Geometry: final body of the model. Coordinates: model frame, mm. Face numbers are marked on the shaded views. Round coordinates to 2 decimals unless told otherwise and drop trailing zeros. Loops run counter-clockwise (first coordinate to the right, second up) from the corner with the lowest first, then second, coordinate; pieces in that order, holes last. Notation, with made-up numbers: M 33,9.25 L 79,9.25 A17 ccw 79,14.25 Z; hole C -9.5,27.25 d2. An arc over 180 degrees is marked long. Answer as a JSON object with one key per item and string values.
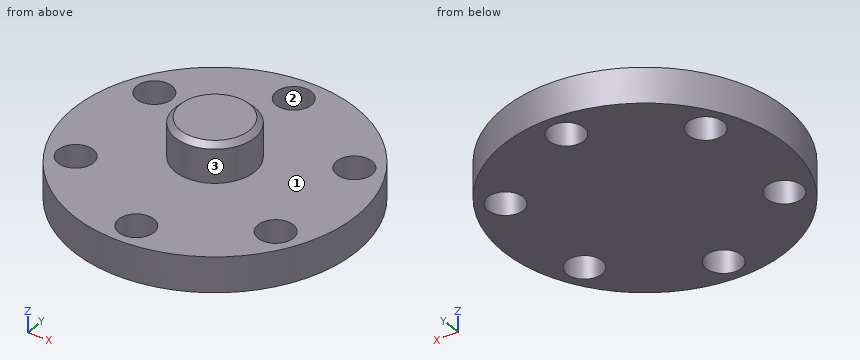
```python
from build123d import *

# Parameters (mm, degrees)
SKETCH1_R               = 80
BASE_EXTRUDE_DEPTH      = 20
CHAMFER1_SIZE           = 3
HOLE_WIZARD_20_0_20_1_D = 20
CIRPATTERN2_COUNT       = 6


with BuildPart() as part:
    # Sketch1 → Base-Extrude (new body)
    with BuildSketch(Plane.XY):
        Circle(SKETCH1_R)
    extrude(amount=BASE_EXTRUDE_DEPTH)

    # Sketch2 → Boss-Revolve1 (revolve)
    with BuildSketch(Plane(origin=(0, 0, 0), x_dir=(1, 0, 0), z_dir=(0, 1, 0))):
        Polygon((-10, -20), (-10, -23), (-22.5, -23), (-22.5, -45), (0, -45), (0, -20), align=None)
    revolve(axis=Axis((0, 0, 0), (0, 0, 1)))

    # Chamfer1
    chamfer1_edges = [part.edges().sort_by_distance(p)[0] for p in [
        (22.5, 0, 45),
    ]]
    chamfer(chamfer1_edges, length=CHAMFER1_SIZE)

    # Ø20.0 (20) 直徑孔1 (through all)
    with Locations(Plane(origin=(0, 65, 20), x_dir=(1, 0, 0), z_dir=(0, 0, 1))):
        with Locations((0, 0)):
            hole_wizard_20_0_20_1 = Hole(HOLE_WIZARD_20_0_20_1_D / 2)

    # CirPattern2: Ø20.0 (20) 直徑孔1 ×6 about axis
    cirpattern2_axis = Axis((0, 0, 0), (0, 0, 1))
    for i in range(1, CIRPATTERN2_COUNT):
        add(hole_wizard_20_0_20_1.rotate(cirpattern2_axis, i * 360 / CIRPATTERN2_COUNT), mode=Mode.SUBTRACT)


solid = part.part
```
1) Cut plane B-B on y = -60. Return the cut outline in (x, z).
Geometry results:
{"outline": "M -52.92,0 L -8.66,0 L -8.66,20 L -52.92,20 Z; M 8.66,0 L 52.92,0 L 52.92,20 L 8.66,20 Z"}
2) First-contact query: pin 1 (6 mm diameter, centred on y = -54.5, z = 21.5, fed in from -X); pin 2 (18 mm diameter, centred on x = 56.29, y = -32.5, fed in from -Z); pin 3 (23 mm diameter, centred on x = 0, y = 65, fed in from +Z); pin 4 (1 mm diameter, centred on x = 4.5, z = 28.5, fed in from +Y). Flat tips, straight axial feed; report the tip coordinate or a pass-through.
Geometry results:
{"pin 1": "x = -60.88", "pin 2": "through", "pin 3": "z = 20", "pin 4": "y = 22.14"}
3) Line query: probe 1 along Y at (x, z) = (0, 11.75); probe 2 along Y at (x, z) = (-58.5, 15); probe 3 along Z at (x, y) = (-18, 5). Output: solid intervals per line, ascending.
Geometry results:
{"probe 1": "-80 to -75, -55 to 55, 75 to 80", "probe 2": "-54.57 to -42.25, -22.75 to 22.75, 42.25 to 54.57", "probe 3": "0 to 20, 23 to 45"}
4) Pull-direction query (Y, two-part tool) for the marked faces 1, 2 and 3; classes: +Y half, -Y half, draft (parallel to the pull), parting line (faces both ways), or undercut.
Geometry results:
{"face 1": "draft", "face 2": "undercut", "face 3": "parting line"}
5) Cut plane A-A on x = 0. Return the cut outline in (y, z).
Geometry results:
{"outline": "M -80,0 L -75,0 L -75,20 L -80,20 Z; M -55,0 L 55,0 L 55,20 L 10,20 L 10,23 L 22.5,23 L 22.5,42 L 19.5,45 L -19.5,45 L -22.5,42 L -22.5,23 L -10,23 L -10,20 L -55,20 Z; M 75,0 L 80,0 L 80,20 L 75,20 Z"}
6) Cut plane D-D on y = 32.5. Return the cut outline in (x, z), and give its area (3 significant figures).
Geometry results:
{"outline": "M -73.1,0 L -66.29,0 L -66.29,20 L -73.1,20 Z; M -46.29,0 L 46.29,0 L 46.29,20 L -46.29,20 Z; M 66.29,0 L 73.1,0 L 73.1,20 L 66.29,20 Z", "area": "2,120 mm2"}
7) Cut plane C-C on z = 11. Return the cut outline in (x, y), and give its area (3 significant figures).
Geometry results:
{"outline": "C 0,0 d160; hole C -56.29,-32.5 d20; hole C -56.29,32.5 d20; hole C 0,-65 d20; hole C 0,65 d20; hole C 56.29,-32.5 d20; hole C 56.29,32.5 d20", "area": "18,200 mm2"}
